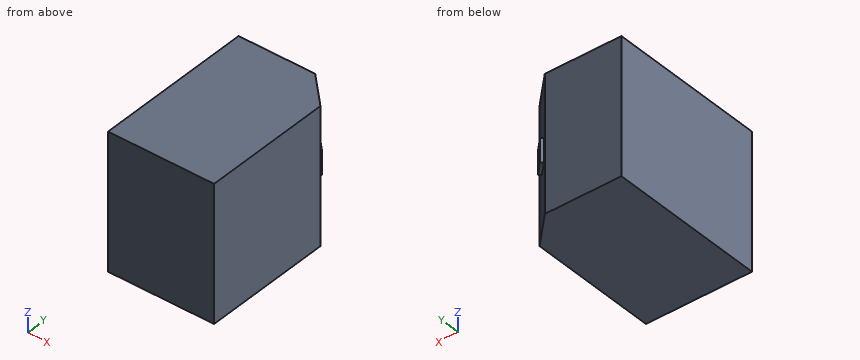
Autodesk Inventor part; units mm, degrees
ref_plane "YZ Plane" through (0, 0, 0) normal (1, 0, 0) x (0, 1, 0)
ref_plane "XZ Plane" through (0, 0, 0) normal (0, 1, 0) x (-1, 0, 0)
ref_plane "XY Plane" through (0, 0, 0) normal (0, 0, 1) x (1, 0, 0)
sketch "Sketch1" plane through (0, 0, 0) normal (0, 1, 0) x (-1, 0, 0)
  line L0 (0, 0) -> (36, 0)
  line L1 (36, 0) -> (36, -46)
  line L2 (36, -46) -> (0, -46)
  line L3 (0, -46) -> (0, 0)
  dimension "d0" = 46
  dimension "d1" = 36
extrude "Extrusion1" add sketch "Sketch1" along normal blind 54
chamfer "Chamfer1" distance 10 angle 45 1 edges at (0, 54, -23)
sketch "Sketch2" plane through (-36, 0, 0) normal (0, 0, 1) x (1, 0, 0)
  point P0 (36, 0)
sketch "Sketch3" plane through (-10, 54, -46) normal (0.7071, 0.7071, 0) x (-0.7071, 0.7071, 0)
  line L0 (-2.5891, 26.7922) -> (-8.0891, 26.7922)
  line L1 (-8.0891, 26.7922) -> (-8.0891, 18.7922)
  line L2 (-8.0891, 18.7922) -> (-2.5891, 18.7922)
  line L3 (-2.5891, 18.7922) -> (-2.5891, 26.7922)
  line L4 (-19.799, 46) -> (18.3848, 46)
  point P0 (-45.2548, 46)
  dimension "d7" = 8
  dimension "d8" = 5.5
extrude "Extrusion2" add sketch "Sketch3" along normal blind 1
sketch "Sketch4" plane through (-10, 54, -46) normal (0.7071, 0.7071, 0) x (-0.7071, 0.7071, 0)
  point P0 (-45.2548, 46)
sketch "Sketch5" plane through (-36, 0, 0) normal (0, 0, 1) x (1, 0, 0)
  point P0 (36, 0)
properties part number "Ventilator"
Build history of the part. All positions in model axes, mm. Round coordinates to 2 decimals unless told otherwise and drop trailing zeros. Loops run counter-clockwise (first coordinate to the right, second up) from the corner with the lowest first, then second, coordinate; pieces in that order, holes last.
Item 1: Saw through at A-A (z = -23.5). List the corners of the cut face in (x, y).
Item 2: Saw through at C-C (z = -18). List the corners of the cut face in (x, y), then the cut area to 3 significant figures.
Item 3: Saw through at B-B (x = -6.5). List the corners of the cut face in (y, z).
Item 4: Pin check, flat tips, straight feed: P1, Ø2.5, axis at x = -5, y = 51.5, coming from the -Z side; P2, Ø1.5, axis at x = -5, z = -21, coming from the +Y side. Stop position of each tip, or through.
Item 5: Drill centre lines: line 1 along X through (y, z) = (48, -8.5); line 2 along Y through (x, z) = (-5, -35); line 3 along Y through (x, z) = (-5, -24.5). Where is each one in solid material? Low to high.
Worked answers:
1. outline: (-36, 0) - (0, 0) - (0, 44) - (-4.28, 48.28) - (-3.57, 48.99) - (-7.46, 52.88) - (-8.17, 52.17) - (-10, 54) - (-36, 54) - close
2. outline: (-36, 0) - (0, 0) - (0, 44) - (-10, 54) - (-36, 54) - close
2. area: 1,890 mm2
3. outline: (0, -46) - (50.5, -46) - (50.5, -27.21) - (51.91, -27.21) - (51.91, -19.21) - (50.5, -19.21) - (50.5, 0) - (0, 0) - close
4. P1: stops at z = -27.21
4. P2: stops at y = 51.16
5. line 1: x = -36 to -4
5. line 2: y = 0 to 49
5. line 3: y = 0 to 50.41
